Geometry check sheet. Reference: drawing and pictorial views, mm from the part's lowest x, y, z. A direction names the side the tool comes from. Coordinates: 2 decimals unless noted, no trailing zeros. Write each loop counter-clockwise with the first axis right and the second up, starting at its lowest first coordinate (ties: lowest second). Pieces come first, ordered by that corner, then holes.
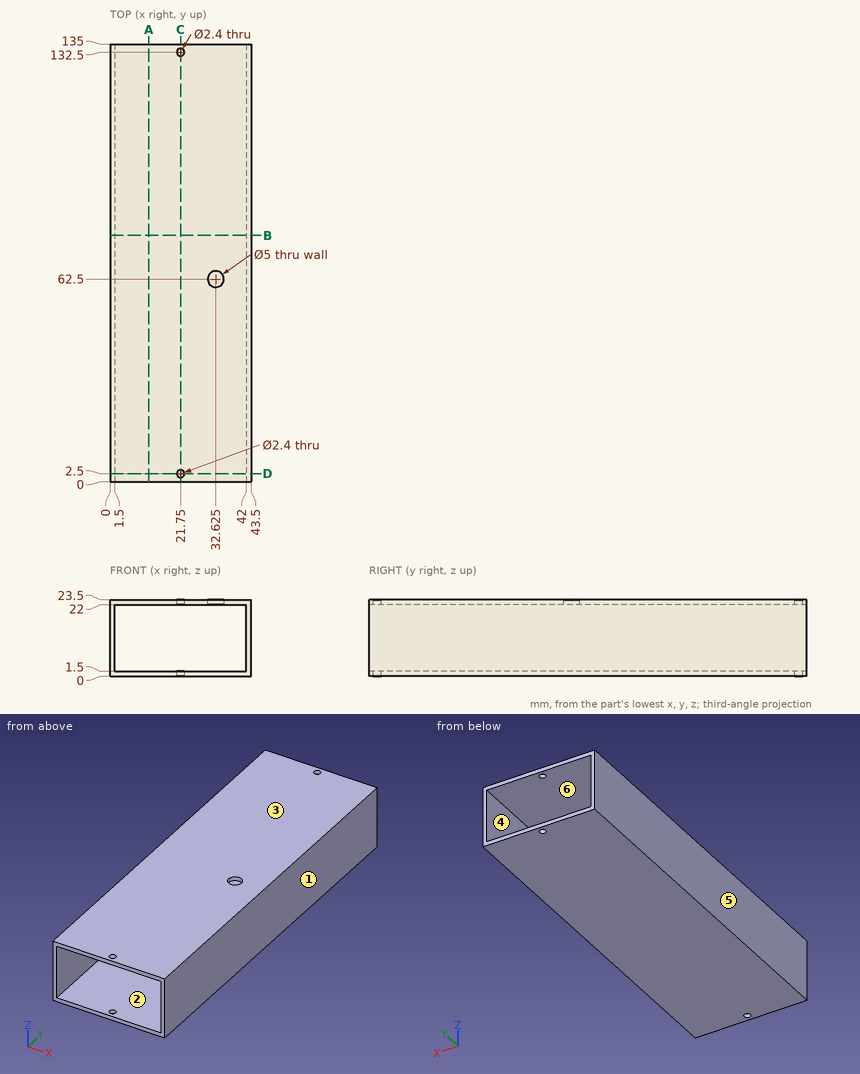
1. Gauge pin test, flat end, axial feed: P1, Ø12, axis at x = 7.5, z = 3.5, coming from the -Y side. Record the tip position at first contact, or that the pin passes through.
2. Sectioned sample at D-D, the plane y = 2.5. Record the boundary of the cut face in (x, z), and give its area (3 significant figures).
3. Draft check along X on the marked faces 1, 2, 3 and 4. Enter one of: pulls with the +X half, pulls with the -X half, needs draft (parallel to the pull), parting line crosses it, or undercut.
4. Material ranges on L1, parallel to Y at x = 21.75, z = 0.4; L2, parallel to X at y = 20, z = 11; L3, parallel to X at y = 132.5, z = 0.5, recorded low to high.
5. Sectioned sample at C-C, the plane x = 21.75. Record the boundary of the cut face in (y, z).
6. Tool access check on the marked faces 5 and 6. Record the directions out of +Z, -Z, +X, -X, +Y, -Y that give a thin tool (end or side, any length) a straight path to the whole face; none if there is none.
7. Sectioned sample at B-B, the plane y = 76. Record the boundary of the cut face in (x, z).
8. Sectioned sample at A-A, the plane x = 12. Record the boundary of the cut face in (y, z), and give its area (3 significant figures).
Outcome:
1. P1: stops at y = 0
2. outline: (0, 0) - (20.55, 0) - (20.55, 1.5) - (1.5, 1.5) - (1.5, 22) - (20.55, 22) - (20.55, 23.5) - (0, 23.5) - close; (22.95, 0) - (43.5, 0) - (43.5, 23.5) - (22.95, 23.5) - (22.95, 22) - (42, 22) - (42, 1.5) - (22.95, 1.5) - close
2. area: 185 mm2
3. face 1: pulls with the +X half
3. face 2: undercut
3. face 3: needs draft
3. face 4: undercut
4. L1: y = 0 to 1.3, 3.7 to 131.3, 133.7 to 135
4. L2: x = 0 to 1.5, 42 to 43.5
4. L3: x = 0 to 20.55, 22.95 to 43.5
5. outline: (0, 0) - (1.3, 0) - (1.3, 1.5) - (0, 1.5) - close; (0, 22) - (1.3, 22) - (1.3, 23.5) - (0, 23.5) - close; (3.7, 0) - (131.3, 0) - (131.3, 1.5) - (3.7, 1.5) - close; (3.7, 22) - (131.3, 22) - (131.3, 23.5) - (3.7, 23.5) - close; (133.7, 0) - (135, 0) - (135, 1.5) - (133.7, 1.5) - close; (133.7, 22) - (135, 22) - (135, 23.5) - (133.7, 23.5) - close
6. face 5: +Z, -Z, -X, +Y, -Y
6. face 6: +Y, -Y
7. outline: (0, 0) - (43.5, 0) - (43.5, 23.5) - (0, 23.5) - close; hole (1.5, 1.5) - (42, 1.5) - (42, 22) - (1.5, 22) - close
8. outline: (0, 0) - (135, 0) - (135, 1.5) - (0, 1.5) - close; (0, 22) - (135, 22) - (135, 23.5) - (0, 23.5) - close
8. area: 405 mm2
